from build123d import *

# Parameters (mm, degrees)
F0_W     = 241.3
F0_H     = 241.3
F1_DEPTH = 38.1
F2_R     = 25.4
F3_R     = 12.7
F5_DEPTH = 19.05
F6_R     = 12.7
F7_DEPTH = 2.54
F8_R     = 12.7
F9_DEPTH = 2.54


with BuildPart() as f1:
    # F0 (on Top) → F1 (new body)
    with BuildSketch(Plane.XY):
        Rectangle(F0_W, F0_H)
    extrude(amount=-F1_DEPTH)

    # F2
    f2_edges = [f1.edges().sort_by_distance(p)[0] for p in [
        (-120.65, -120.65, -19.05),
        (-120.65, 120.65, -19.05),
        (120.65, 120.65, -19.05),
        (120.65, -120.65, -19.05),
    ]]
    fillet(f2_edges, radius=F2_R)

    # F3
    f3_edges = [f1.edges().sort_by_distance(p)[0] for p in [
        (0, -120.65, -38.1),
    ]]
    fillet(f3_edges, radius=F3_R)

    # F4 (on face) → F5 (cut)
    with BuildSketch(Plane(origin=(0, 0, -38.1), x_dir=(1, 0, 0), z_dir=(0, 0, -1))):
        with BuildLine():
            Line((-28.575, -20.163958), (-3.175, -34.828655))
            ThreePointArc((-3.175, -34.828655), (0, -35.679394), (3.175, -34.828655))
            Line((3.175, -34.828655), (28.575, -20.163958))
            ThreePointArc((28.575, -20.163958), (30.899261, -17.839697), (31.75, -14.664697))
            Line((31.75, -14.664697), (31.75, 14.664697))
            ThreePointArc((31.75, 14.664697), (30.899261, 17.839697), (28.575, 20.163958))
            Line((28.575, 20.163958), (3.175, 34.828655))
            ThreePointArc((3.175, 34.828655), (0, 35.679394), (-3.175, 34.828655))
            Line((-3.175, 34.828655), (-28.575, 20.163958))
            ThreePointArc((-28.575, 20.163958), (-30.899261, 17.839697), (-31.75, 14.664697))
            Line((-31.75, 14.664697), (-31.75, -14.664697))
            ThreePointArc((-31.75, -14.664697), (-30.899261, -17.839697), (-28.575, -20.163958))
        make_face()
    extrude(amount=-F5_DEPTH, mode=Mode.SUBTRACT)

    # F6 (on face) → F7 (cut)
    with BuildSketch(Plane.XY):
        with Locations((-101.6, 0)):
            Circle(F6_R)
    extrude(amount=-F7_DEPTH, mode=Mode.SUBTRACT)

    # F8 (on face) → F9 (cut)
    with BuildSketch(Plane.XY):
        Circle(F8_R)
    extrude(amount=-F9_DEPTH, mode=Mode.SUBTRACT)


solid = f1.part
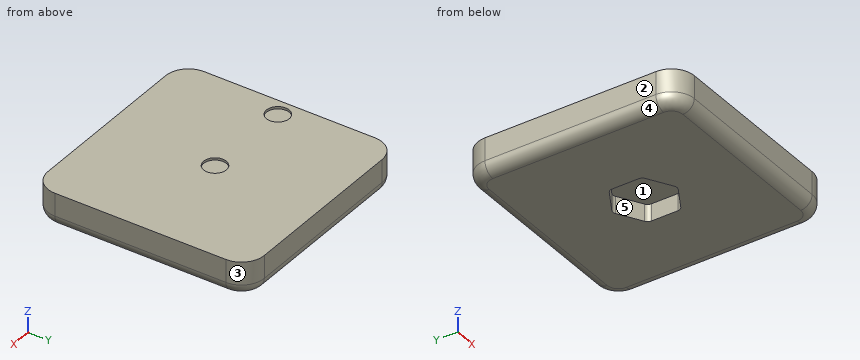
Source: CAD feature listing. Evaluate the final solid. Frame: model axes, mm. Face numbers are marked on the shaded views. A direction names the side the tool comes from. Round coordinates to 2 decimals unless told otherwise and drop trailing zeros. Loops run counter-clockwise (first coordinate to the right, second up) from the corner with the lowest first, then second, coordinate; pieces in that order, holes last. Notation, with made-up numbers: (45.5, 85) - (104.5, 85) arc R31 ccw to (104.5, 114) - close; hole circle Ø11 at (15.25, 47). An arc over 180 degrees is marked (long way). Write item = value, one per line. Start each with the question number.
Item 1: Section query C-C on y = -28. Output: boundary loops of the cut face in (x, z), plus the area to 3 significant figures.
Item 2: Material intervals for line 1 (Y direction, x = 0, z = -1.7); line 2 (Z direction, x = -6, y = -20); line 3 (Z direction, x = -108.5, y = -11.5), sorted ascending.
Item 3: Reachability of the marked faces 1 and 2 from +Z, -Z, +X, -X, +Y, -Y: full face, straight path, thin tool, end or side. Return the list, or none.
Item 4: Mould query, pull axis Y, two halves, no side actions, for the marked faces 3, 4 and 5. Classes: released by +Y, released by -Y, zero draft, split by the parting line, or undercut.
Item 5: Section query D-D on y = 27.5. Output: boundary loops of the cut face in (x, z), plus the area to 3 significant figures.
Item 6: Section query A-A on x = 0. Output: boundary loops of the cut face in (y, z).
Item 7: First-contact query: pin 1 Ø15 at (x, y) = (-101.6, 0) entering from +Z; pin 2 Ø1 at (y, z) = (33.5, -27.5) entering from -X. Flat tips, straight axial feed; report the tip coordinate or a pass-through.
Item 8: Section query B-B on y = 0. Output: boundary loops of the cut face in (x, z), plus the area to 3 significant figures.
Results list:
q1.outline = (-120.65, -25.4) arc R12.7 ccw to (-107.95, -38.1) - (-15, -38.1) - (-15, -19.05) - (15, -19.05) - (15, -38.1) - (107.95, -38.1) arc R12.7 ccw to (120.65, -25.4) - (120.65, 0) - (-120.65, 0) - close
q1.area = 8,550 mm²
q2.line_1 = -120.65 to -12.7, 12.7 to 120.65
q2.line_2 = -19.05 to 0
q2.line_3 = -38.09 to 0
q3.face_1 = -Z
q3.face_2 = +Z, -Z, -X, +Y, -Y
q4.face_3 = released by +Y
q4.face_4 = zero draft
q4.face_5 = undercut
q5.outline = (-120.65, -25.4) arc R12.7 ccw to (-107.95, -38.1) - (-15.87, -38.1) - (-15.87, -19.05) - (15.87, -19.05) - (15.87, -38.1) - (107.95, -38.1) arc R12.7 ccw to (120.65, -25.4) - (120.65, 0) - (-120.65, 0) - close
q5.area = 8,520 mm²
q6.outline = (-120.65, -25.4) arc R12.7 ccw to (-107.95, -38.1) - (-35.68, -38.1) - (-35.68, -19.05) - (35.68, -19.05) - (35.68, -38.1) - (107.95, -38.1) arc R12.7 ccw to (120.65, -25.4) - (120.65, 0) - (12.7, 0) - (12.7, -2.54) - (-12.7, -2.54) - (-12.7, 0) - (-120.65, 0) - close
q7.pin_1 = -2.54
q7.pin_2 = -120.55
q8.outline = (-120.65, -25.4) arc R12.7 ccw to (-107.95, -38.1) - (-31.75, -38.1) - (-31.75, -19.05) - (31.75, -19.05) - (31.75, -38.1) - (107.95, -38.1) arc R12.7 ccw to (120.65, -25.4) - (120.65, 0) - (12.7, 0) - (12.7, -2.54) - (-12.7, -2.54) - (-12.7, 0) - (-88.9, 0) - (-88.9, -2.54) - (-114.3, -2.54) - (-114.3, 0) - (-120.65, 0) - close
q8.area = 7,790 mm²
